Autodesk Inventor part; units mm, degrees
ref_plane "YZ Plane" through (0, 0, 0) normal (1, 0, 0) x (0, 1, 0)
ref_plane "XZ Plane" through (0, 0, 0) normal (0, 1, 0) x (-1, 0, 0)
ref_plane "XY Plane" through (0, 0, 0) normal (0, 0, 1) x (1, 0, 0)
sketch "Sketch1" plane through (0, 0, 0) normal (0, 1, 0) x (-1, 0, 0)
  line L0 (47.625, 47.625) -> (-47.625, 47.625)
  line L1 (-47.625, 47.625) -> (-47.625, -47.625)
  line L2 (-47.625, -47.625) -> (47.625, -47.625)
  line L3 (47.625, -47.625) -> (47.625, 47.625)
  line L4 (47.625, 47.625) -> (-47.625, -47.625) construction
  line L5 (-47.625, 47.625) -> (47.625, -47.625) construction
  point P0 (0, 0)
  dimension "d0" = 95.25
extrude "Extrusion1" add sketch "Sketch1" against normal blind 6.35
sketch "Sketch2" plane through (0, 0, 0) normal (0, 1, 0) x (1, 0, 0)
  line L0 (-25.4, -12.7) -> (25.4, -12.7)
  line L1 (25.4, -12.7) -> (25.4, 12.7)
  line L2 (25.4, 12.7) -> (-25.4, 12.7)
  line L3 (-25.4, 12.7) -> (-25.4, -12.7)
  line L4 (-25.4, -12.7) -> (25.4, 12.7) construction
  line L5 (25.4, -12.7) -> (-25.4, 12.7) construction
  line L6 (-22.225, -9.525) -> (22.225, -9.525)
  line L7 (22.225, -9.525) -> (22.225, 9.525)
  line L8 (22.225, 9.525) -> (-22.225, 9.525)
  line L9 (-22.225, 9.525) -> (-22.225, -9.525)
  line L10 (-22.225, -9.525) -> (22.225, 9.525) construction
  line L11 (22.225, -9.525) -> (-22.225, 9.525) construction
  point P0 (0, 0)
  dimension "d3" = 50.8
  dimension "d4" = 25.4
  dimension "d5" = 3.175
  dimension "d6" = 3.175
extrude "Extrusion2" add sketch "Sketch2" along normal blind 152.4
sketch "Sketch3" plane through (-25.4, 0, 12.7) normal (0, 0, 1) x (1, 0, 0)
  line L0 (25.4, 0) -> (25.4, 152.4) construction
  line L1 (0, 152.4) -> (50.8, 152.4) construction
  line L2 (-22.225, 0) -> (73.025, 0) construction
  point P0 (25.4, 101.6)
  dimension "d9" = 101.6
hole "Hole1" at (0, 101.6, 12.7) direction (0, 0, -1) diameter 31.75 end up to surface
sketch "Sketch4" plane through (25.4, 0, -12.7) normal (0, 0, -1) x (-1, 0, 0)
  line L0 (25.4, 0) -> (25.4, 152.4) construction
  line L1 (50.8, 152.4) -> (0, 152.4) construction
  circle A0 centre (25.4, 101.6) radius 15.875
hole "Hole2" at (0, 101.6, -12.7) direction (0, 0, 1) diameter 13.7414 end up to surface
sketch "Sketch5" plane through (0, 0, 0) normal (0, 1, 0) x (1, 0, 0)
  line L0 (-34.925, -34.925) -> (34.925, -34.925) construction
  line L1 (34.925, -34.925) -> (34.925, 34.925) construction
  line L2 (34.925, 34.925) -> (-34.925, 34.925) construction
  line L3 (-34.925, 34.925) -> (-34.925, -34.925) construction
  line L4 (-34.925, -34.925) -> (34.925, 34.925) construction
  line L5 (34.925, -34.925) -> (-34.925, 34.925) construction
  line L6 (-47.625, 47.625) -> (-47.625, -47.625)
  line L7 (47.625, 47.625) -> (-47.625, 47.625)
  point P0 (0, 0)
  dimension "d25" = 12.7
  dimension "d26" = 12.7
hole "Hole3" at (-34.925, 0, -34.925) at (34.925, 0, -34.925) at (34.925, 0, 34.925) at (-34.925, 0, 34.925) direction (0, -1, 0) diameter 6.7564 end through all
equation "\"d1\" = baseMaterialThickness"
equation "\"d5\" = postMaterialThickness"
equation "\"d6\" = postMaterialThickness"
equation "\"d10\" = flangeBearingHoleDiam"
equation "\"flangeBearingHoleDiam\" = 31.75"
equation "\"heightOfRod\" = 101.6"
equation "\"hightOfPost\" = 152.4"
equation "\"postMaterialThickness\" = 3.175"
equation "\"baseMaterialThickness\" = 6.35"
properties part number "ThunderhexPost"
The listing builds one solid part. Answer for the finished solid, in the listing's coordinates (mm). A direction names the side the tool comes from. Coordinates: 2 decimals unless noted, no trailing zeros. Write each loop counter-clockwise with the first axis right and the second up, starting at its lowest first coordinate (ties: lowest second). Pieces come first, ordered by that corner, then holes. Notation, with made-up numbers: (59.25, -31) -> (78.25, -31) arc R7 cw to (78.25, -21) -> close; hole circle Ø6 at (-18.75, 26.25). An arc over 180 degrees is marked (long way). Write each question's results on one line, items separated by ' | '. Start each with the question number.
1) For a pull along Y with two mould halves and no side action, classify faces 4 (the flat face through (0, 75, 12.7)), 5 (the flat face through (0, 152.4, -10)), 6 (the cylindrical face through (4.181, 96.148, -11.09)) as +Y half, -Y half, draft (parallel to the pull), parting line (faces both ways), or undercut.
2) Straight lines are drawn through the part: probe 1 along X at (y, z) = (101, 10); probe 2 along Z at (x, y) = (-11.5, 50) (3 decimals); probe 3 along X at (y, z) = (101.6, -10.5). For each, find the intervals that lie inside material, in ascending order.
3) A cutting plane is placed at B-B (y = 62). Determine the outline of the cut face in (x, z) (3 decimals).
4) A cutting plane is placed at C-C (y = 101.6). Determine the outline of the cut face in (x, z) (3 decimals).
5) A tool of negligible diameter and unlimited length cuts with its end or side. For faces 1 (the cylindrical face through (-0.7, 117.46, 11.09)), 2 (the flat face through (0, 75, -12.7)), 3 (the flat face through (0, 0, 0)), from which of +Z, -Z, +X, -X, +Y, -Y can it reach the whole face along a straight path? Write none if from no direction.
6) Flat-ended cylindrical pins translate along their axes: pin 1 Ø21 at (y, z) = (45, 2.5) entering from +X; pin 2 Ø13.5 at (x, y) = (8.5, 76) entering from +Z; pin 3 Ø15 at (x, y) = (-3, 104) entering from -Z. Find the tip coordinate at first contact, or state that the pin passes through.
7) A cutting plane is placed at D-D (z = -4). Determine the outline of the cut face in (x, y) (3 decimals).
8) A cutting plane is placed at A-A (x = 0). Determine the outline of the cut face in (y, z) (3 decimals), then the cut area to 3 significant figures.
Values follow:
1) face 4: draft | face 5: +Y half | face 6: undercut
2) probe 1: -25.4 to -15.86, 15.86 to 25.4 | probe 2: -12.7 to -9.525, 9.525 to 12.7 | probe 3: -25.4 to -6.87, 6.87 to 25.4
3) outline: (-25.4, -12.7) -> (25.4, -12.7) -> (25.4, 12.7) -> (-25.4, 12.7) -> close; hole (-22.225, -9.525) -> (22.225, -9.525) -> (22.225, 9.525) -> (-22.225, 9.525) -> close
4) outline: (-25.4, -12.7) -> (-6.871, -12.7) -> (-6.871, -9.525) -> (-22.225, -9.525) -> (-22.225, 9.525) -> (-15.875, 9.525) -> (-15.875, 12.7) -> (-25.4, 12.7) -> close; (6.871, -12.7) -> (25.4, -12.7) -> (25.4, 12.7) -> (15.875, 12.7) -> (15.875, 9.525) -> (22.225, 9.525) -> (22.225, -9.525) -> (6.871, -9.525) -> close
5) face 1: +Z | face 2: -Z, +X, -X, +Y | face 3: +Y
6) pin 1: x = 25.4 | pin 2: z = 12.7 | pin 3: z = -12.7
7) outline: (-47.625, -6.35) -> (47.625, -6.35) -> (47.625, 0) -> (25.4, 0) -> (25.4, 152.4) -> (22.225, 152.4) -> (22.225, 0) -> (-22.225, 0) -> (-22.225, 152.4) -> (-25.4, 152.4) -> (-25.4, 0) -> (-47.625, 0) -> close
8) outline: (-6.35, -47.625) -> (0, -47.625) -> (0, -12.7) -> (94.729, -12.7) -> (94.729, -9.525) -> (0, -9.525) -> (0, 9.525) -> (85.725, 9.525) -> (85.725, 12.7) -> (0, 12.7) -> (0, 47.625) -> (-6.35, 47.625) -> close; (108.471, -12.7) -> (152.4, -12.7) -> (152.4, -9.525) -> (108.471, -9.525) -> close; (117.475, 9.525) -> (152.4, 9.525) -> (152.4, 12.7) -> (117.475, 12.7) -> close | area: 1,430 mm²
